```python
from build123d import *

# Parameters (mm, degrees)
SCHIZZO1_W                   = 31
SCHIZZO1_H                   = 31
SCHIZZO1_W_2                 = 26
SCHIZZO1_H_2                 = 26
ESTRUSIONE_SOTTILE1_DEPTH    = 8
SCHIZZO2_W                   = 31
SCHIZZO2_H                   = 31
ESTRUSIONE_ESTRUSIONE1_DEPTH = 2
RACCORDO1_R                  = 2.5
RACCORDO2_R                  = 0.4
TAGLIO_ESTRUSIONE1_REACH     = 37.57
SCHIZZO3_R                   = 1.5


with BuildPart() as part:
    # Schizzo1 → Estrusione-Sottile1 (new body)
    with BuildSketch(Plane.XY):
        Rectangle(SCHIZZO1_W, SCHIZZO1_H)
        Rectangle(SCHIZZO1_W_2, SCHIZZO1_H_2, mode=Mode.SUBTRACT)
    extrude(amount=ESTRUSIONE_SOTTILE1_DEPTH)

    # Schizzo2 → Estrusione-Estrusione1 (add)
    with BuildSketch(Plane(origin=(0, 0, 0), x_dir=(-1, 0, 0), z_dir=(0, 0, -1))):
        Rectangle(SCHIZZO2_W, SCHIZZO2_H)
    extrude(amount=ESTRUSIONE_ESTRUSIONE1_DEPTH)

    # Raccordo1
    raccordo1_edges = [part.edges().sort_by_distance(p)[0] for p in [
        (-15.5, 15.5, 3),
        (15.5, 15.5, 3),
        (15.5, -15.5, 3),
        (-15.5, -15.5, 3),
    ]]
    fillet(raccordo1_edges, radius=RACCORDO1_R)

    # Raccordo2
    raccordo2_edges = [part.edges().sort_by_distance(p)[0] for p in [
        (-13, 0, 0),
        (-13, 13, 4),
        (0, -13, 0),
        (-13, -13, 4),
        (13, 0, 0),
        (13, -13, 4),
        (0, 13, 0),
        (13, 13, 4),
    ]]
    fillet(raccordo2_edges, radius=RACCORDO2_R)

    # Schizzo3 → Taglio-Estrusione1 (cut, up to next)
    with BuildSketch(Plane.ZY.offset(15.5), mode=Mode.PRIVATE) as taglio_estrusione1_sk1:
        with Locations((8, -9.5)):
            Circle(SCHIZZO3_R)
    taglio_estrusione1_tool1 = extrude(taglio_estrusione1_sk1.sketch, amount=-TAGLIO_ESTRUSIONE1_REACH, mode=Mode.PRIVATE) & part.part
    add(taglio_estrusione1_tool1.solids().sort_by_distance((-15.5, -9.5, 8))[0], mode=Mode.SUBTRACT)


solid = part.part
```
Design review of the part built by this model. Coordinates are the model's own, in mm. A direction names the side the tool comes from. Give positions to 0.01 mm unless a question says otherwise; leave off trailing zeros. Order: outer loops, then holes, each group sorted by start corner. A loop starts at its lowest first (then second) coordinate and runs counter-clockwise, first axis right, second up. Notation, with made-up numbers: (52, 48.5) - (111, 48.5) arc R20 ccw to (111, 86.5) - close; hole circle Ø7 at (86, 45.25). An arc over 180 degrees is marked (long way). Use a Markdown table: item, result. Add a question column.
(1) Wall thickness on probe 1 along X at (y, z) = (10, 1.25); probe 2 along Z at (x, y) = (-7.5, -11.5): over which ranges is each line inside the solid? List them lowest first. Write a range as [from, to].
(2) Mouldability with a two-part tool opening along Y and no side actions: class faces 1 (the face through (14, 0, 8)), 2 (the face through (13, 0, 4)), 3 (the face through (14.787, 14.748, 3.07)) as +Y half, -Y half, draft (parallel to the pull), parting line (faces both ways), or undercut.
(3) Machinability: for faces 4 (the face through (0, 13, 4)), 5 (the face through (-14.3, -9.5, 6.5)), 6 (the face through (0, -15.5, 3)), which of the approach directions +Z, -Z, +X, -X, +Y, -Y give a long, thin tool a straight path to every point of the face, cutting with its end or side? Answer none if there is none.
(4) Add section A-A on x = 5. Give the boundary of the cut face in (y, z), then the cut area to 3 significant figures.
(5) Clearance check with a flat-ended pin moving along its axis: P1, Ø3, axis at x = 10, y = -7, coming from the +Z side. State where the tip first meets the part, or that it passes through.
(6) Add section C-C on z = 7.25. Give the boundary of the cut face in (x, y), then the cut area to 3 significant figures.
(7) Add section B-B on y = -9.5. Give the boundary of the cut face in (x, z), then the cut area to 3 significant figures.
Report:
| question | item | result |
|---|---|---|
| 1 | probe 1 | x = [-15.5, -13], [13, 15.5] |
| 1 | probe 2 | z = [-2, 0] |
| 2 | face 1 | draft |
| 2 | face 2 | undercut |
| 2 | face 3 | +Y half |
| 3 | face 4 | +Z |
| 3 | face 5 | +Z, -X |
| 3 | face 6 | +Z, -Z, +X, -X, -Y |
| 4 | outline | (-15.5, -2) - (15.5, -2) - (15.5, 8) - (13, 8) - (13, 0.4) arc R0.4 cw to (12.6, 0) - (-12.6, 0) arc R0.4 cw to (-13, 0.4) - (-13, 8) - (-15.5, 8) - close |
| 4 | area | 102 mm² |
| 5 | P1 | stops at z = 0 |
| 6 | outline | (-15.5, -13) arc R2.5 ccw to (-13, -15.5) - (13, -15.5) arc R2.5 ccw to (15.5, -13) - (15.5, 13) arc R2.5 ccw to (13, 15.5) - (-13, 15.5) arc R2.5 ccw to (-15.5, 13) - (-15.5, -8.2) - (-13, -8.2) - (-13, 12.6) arc R0.4 cw to (-12.6, 13) - (12.6, 13) arc R0.4 cw to (13, 12.6) - (13, -12.6) arc R0.4 cw to (12.6, -13) - (-12.6, -13) arc R0.4 cw to (-13, -12.6) - (-13, -10.8) - (-15.5, -10.8) - close |
| 6 | area | 273 mm² |
| 7 | outline | (-15.5, -2) - (15.5, -2) - (15.5, 8) - (13, 8) - (13, 0.4) arc R0.4 cw to (12.6, 0) - (-12.6, 0) arc R0.4 cw to (-13, 0.4) - (-13, 6.5) - (-15.5, 6.5) - close |
| 7 | area | 98.3 mm² |
